The model under review builds one solid part; all positions refer to its coordinate system, in mm. A direction names the side the tool comes from. Coordinates: 2 decimals unless noted, no trailing zeros. Write each loop counter-clockwise with the first axis right and the second up, starting at its lowest first coordinate (ties: lowest second). Pieces come first, ordered by that corner, then holes.
```python
from build123d import *

# Parameters (mm, degrees)
F0_W         = 85
F0_H         = 44
F1_DEPTH     = 28
F2_W         = 49
F2_H         = 37
F3_DEPTH     = 9
F2_W_2       = 25
F2_H_2       = 42
F4_DEPTH     = 7.5
F5_W         = 25
F5_H         = 13
F5_R         = 1.25
F6_DEPTH     = 16
F7_T1_DEPTH  = 22
F7_T3_DEPTH  = 32.5
F7_T5_DEPTH  = 79
F7_T7_DEPTH  = 38
F7_T9_DEPTH  = 68
F7_T11_DEPTH = 89.5
F7_T13_DEPTH = 48.5
F7_S17_W     = 3
F7_S17_H     = 3
F7_T18_DEPTH = 3
F7_S23_W     = 3
F7_S23_H     = 3
F7_T24_DEPTH = 3
F7_S29_W     = 3
F7_S29_H     = 3
F7_T30_DEPTH = 3
F7_S35_W     = 3
F7_S35_H     = 3
F7_T36_DEPTH = 3
F7_S41_W     = 3
F7_S41_H     = 3
F7_T42_DEPTH = 3


# Not quite as in the source:
# - a fillet or chamfer that OpenCascade refuses, or shapes differently, is made with other operations: its cross-section is extruded or revolved along the edge and cut away or added


with BuildPart() as f1:
    # F0 (on Top) → F1 (new body)
    with BuildSketch(Plane.XY):
        with Locations((12.7505162358, -9.2363715138)):
            Rectangle(F0_W, F0_H)
    extrude(amount=F1_DEPTH)

    # F2 (on face) → F3 (cut)
    with BuildSketch(Plane.XY.offset(28)):
        with Locations((-3.2494837642, -9.2363715138)):
            Rectangle(F2_W, F2_H)
    extrude(amount=-F3_DEPTH, mode=Mode.SUBTRACT)

    # F2 (on face) → F4 (cut)
    with BuildSketch(Plane.XY.offset(28)):
        with Locations((35.7505162358, -8.2363715138)):
            Rectangle(F2_W_2, F2_H_2)
    extrude(amount=-F4_DEPTH, mode=Mode.SUBTRACT)

    # F5 (on face) → F6 (cut)
    with BuildSketch(Plane(origin=(0, 0, 0), x_dir=(1, 0, 0), z_dir=(0, 0, -1))):
        with Locations((-12.2494837642, 9.2363715138)):
            Rectangle(F5_W, F5_H)
        with Locations((37.7505162358, 9.2363715138)):
            Rectangle(F5_W, F5_H)
        with Locations((-26.9994837642, 9.2363715138)):
            Circle(F5_R)
        with Locations((2.5005162358, 9.2363715138)):
            Circle(F5_R)
        with Locations((23.0005162358, 9.2363715138)):
            Circle(F5_R)
        with Locations((52.5005162358, 9.2363715138)):
            Circle(F5_R)
    extrude(amount=-F6_DEPTH, mode=Mode.SUBTRACT)

    # F7: fillet of radius 3 on 11 edges, made by hand

    # F7_s2 → F7_t1 (cut)
    with BuildSketch(Plane.XY.offset(3)):
        with BuildLine():
            ThreePointArc((55.2505162358, -28.2363715138), (54.3718365794, -30.3576918574), (52.2505162358, -31.2363715138))
            Line((52.2505162358, -31.2363715138), (55.2505162358, -31.2363715138))
            Line((55.2505162358, -31.2363715138), (55.2505162358, -28.2363715138))
        make_face()
    extrude(amount=F7_T1_DEPTH, mode=Mode.SUBTRACT)

    # F7_s4 → F7_t3 (cut)
    with BuildSketch(Plane.XY.offset(3)):
        with BuildLine():
            ThreePointArc((52.2505162358, 12.7636284862), (54.3718365794, 11.8849488297), (55.2505162358, 9.7636284862))
            Line((55.2505162358, 9.7636284862), (55.2505162358, 12.7636284862))
            Line((55.2505162358, 12.7636284862), (52.2505162358, 12.7636284862))
        make_face()
        with BuildLine():
            ThreePointArc((-29.7494837642, -28.2363715138), (-28.8708041077, -30.3576918574), (-26.7494837642, -31.2363715138))
            Line((-26.7494837642, -31.2363715138), (-29.7494837642, -31.2363715138))
            Line((-29.7494837642, -31.2363715138), (-29.7494837642, -28.2363715138))
        make_face()
        with BuildLine():
            ThreePointArc((-26.7494837642, 12.7636284862), (-28.8708041077, 11.8849488297), (-29.7494837642, 9.7636284862))
            Line((-29.7494837642, 9.7636284862), (-29.7494837642, 12.7636284862))
            Line((-29.7494837642, 12.7636284862), (-26.7494837642, 12.7636284862))
        make_face()
    extrude(amount=F7_T3_DEPTH, mode=Mode.SUBTRACT)

    # F7_s6 → F7_t5 (cut)
    with BuildSketch(Plane.YZ.offset(-26.7494837642)):
        with BuildLine():
            ThreePointArc((12.7636284862, 3), (11.8849488297, 0.8786796564), (9.7636284862, 0))
            Line((9.7636284862, 0), (12.7636284862, 0))
            Line((12.7636284862, 0), (12.7636284862, 3))
        make_face()
        with BuildLine():
            ThreePointArc((-28.2363715138, 0), (-30.3576918574, 0.8786796564), (-31.2363715138, 3))
            Line((-31.2363715138, 3), (-31.2363715138, 0))
            Line((-31.2363715138, 0), (-28.2363715138, 0))
        make_face()
    extrude(amount=F7_T5_DEPTH, mode=Mode.SUBTRACT)

    # F7_s8 → F7_t7 (cut)
    with BuildSketch(Plane.XZ.offset(-9.7636284862)):
        with BuildLine():
            ThreePointArc((-26.7494837642, 0), (-28.8708041077, 0.8786796564), (-29.7494837642, 3))
            Line((-29.7494837642, 3), (-29.7494837642, 0))
            Line((-29.7494837642, 0), (-26.7494837642, 0))
        make_face()
        with BuildLine():
            ThreePointArc((52.2505162358, 0), (54.3718365794, 0.8786796564), (55.2505162358, 3))
            Line((55.2505162358, 3), (55.2505162358, 0))
            Line((55.2505162358, 0), (52.2505162358, 0))
        make_face()
    extrude(amount=F7_T7_DEPTH, mode=Mode.SUBTRACT)

    # F7_s10 → F7_t9 (cut)
    with BuildSketch(Plane.YZ.offset(-37.2494837642)):
        with BuildLine():
            ThreePointArc((12.7636284862, 25), (11.8849488297, 27.1213203436), (9.7636284862, 28))
            Line((9.7636284862, 28), (12.7636284862, 28))
            Line((12.7636284862, 28), (12.7636284862, 25))
        make_face()
    extrude(amount=F7_T9_DEPTH, mode=Mode.SUBTRACT)

    # F7_s12 → F7_t11 (cut)
    with BuildSketch(Plane.YZ.offset(-37.2494837642)):
        with BuildLine():
            ThreePointArc((-28.2363715138, 28), (-30.3576918574, 27.1213203436), (-31.2363715138, 25))
            Line((-31.2363715138, 25), (-31.2363715138, 28))
            Line((-31.2363715138, 28), (-28.2363715138, 28))
        make_face()
    extrude(amount=F7_T11_DEPTH, mode=Mode.SUBTRACT)

    # F7_s14 → F7_t13 (cut)
    with BuildSketch(Plane.XZ.offset(-20.2636284862)):
        with BuildLine():
            ThreePointArc((52.2505162358, 28), (54.3718365794, 27.1213203436), (55.2505162358, 25))
            Line((55.2505162358, 25), (55.2505162358, 28))
            Line((55.2505162358, 28), (52.2505162358, 28))
        make_face()
    extrude(amount=F7_T13_DEPTH, mode=Mode.SUBTRACT)


with BuildPart() as f7_tool16:
    # F7_s17 → F7_t18 (new body)
    with BuildSketch(Plane.XZ.offset(28.2363715138)):
        with Locations((53.7505162358, 1.5)):
            Rectangle(F7_S17_W, F7_S17_H)
    extrude(amount=F7_T18_DEPTH)

    # F7_s19 → F7_t20 (revolve, cut)
    with BuildSketch(Plane(origin=(52.2505162358, -28.2363715138, 3), x_dir=(-0.7071067812, 0, 0.7071067812), z_dir=(0.7071067812, 0, 0.7071067812))):
        with BuildLine():
            ThreePointArc((0, -3), (3, 0), (0, 3))
            Line((0, 3), (0, -3))
        make_face()
    revolve(axis=Axis((52.2505162358, -28.2363715138, 3), (0, -1, 0)), mode=Mode.SUBTRACT)


with BuildPart() as f1_1:
    add(f1.part)

    # F7_t15: cut F7_tool16
    add(f7_tool16.part, mode=Mode.SUBTRACT)


with BuildPart() as f7_tool22:
    # F7_s23 → F7_t24 (new body)
    with BuildSketch(Plane.XZ.offset(28.2363715138)):
        with Locations((53.7505162358, 26.5)):
            Rectangle(F7_S23_W, F7_S23_H)
    extrude(amount=F7_T24_DEPTH)

    # F7_s25 → F7_t26 (revolve, cut)
    with BuildSketch(Plane(origin=(52.2505162358, -28.2363715138, 25), x_dir=(-0.7071067812, 0, -0.7071067812), z_dir=(-0.7071067812, 0, 0.7071067812))):
        with BuildLine():
            ThreePointArc((0, -3), (3, 0), (0, 3))
            Line((0, 3), (0, -3))
        make_face()
    revolve(axis=Axis((52.2505162358, -28.2363715138, 25), (0, -1, 0)), mode=Mode.SUBTRACT)


with BuildPart() as f1_2:
    add(f1_1.part)

    # F7_t21: cut F7_tool22
    add(f7_tool22.part, mode=Mode.SUBTRACT)


with BuildPart() as f7_tool28:
    # F7_s29 → F7_t30 (new body)
    with BuildSketch(Plane.XZ.offset(-9.7636284862)):
        with Locations((53.7505162358, 1.5)):
            Rectangle(F7_S29_W, F7_S29_H)
    extrude(amount=-F7_T30_DEPTH)

    # F7_s31 → F7_t32 (revolve, cut)
    with BuildSketch(Plane(origin=(52.2505162358, 9.7636284862, 3), x_dir=(-0.7071067812, 0, 0.7071067812), z_dir=(-0.7071067812, 0, -0.7071067812))):
        with BuildLine():
            ThreePointArc((0, -3), (3, 0), (0, 3))
            Line((0, 3), (0, -3))
        make_face()
    revolve(axis=Axis((52.2505162358, 9.7636284862, 3), (0, 1, 0)), mode=Mode.SUBTRACT)


with BuildPart() as f1_3:
    add(f1_2.part)

    # F7_t27: cut F7_tool28
    add(f7_tool28.part, mode=Mode.SUBTRACT)


with BuildPart() as f7_tool34:
    # F7_s35 → F7_t36 (new body)
    with BuildSketch(Plane.XZ.offset(28.2363715138)):
        with Locations((-28.2494837642, 1.5)):
            Rectangle(F7_S35_W, F7_S35_H)
    extrude(amount=F7_T36_DEPTH)

    # F7_s37 → F7_t38 (revolve, cut)
    with BuildSketch(Plane(origin=(-26.7494837642, -28.2363715138, 3), x_dir=(0.7071067812, 0, 0.7071067812), z_dir=(0.7071067812, 0, -0.7071067812))):
        with BuildLine():
            ThreePointArc((0, -3), (3, 0), (0, 3))
            Line((0, 3), (0, -3))
        make_face()
    revolve(axis=Axis((-26.7494837642, -28.2363715138, 3), (0, -1, 0)), mode=Mode.SUBTRACT)


with BuildPart() as f1_4:
    add(f1_3.part)

    # F7_t33: cut F7_tool34
    add(f7_tool34.part, mode=Mode.SUBTRACT)


with BuildPart() as f7_tool40:
    # F7_s41 → F7_t42 (new body)
    with BuildSketch(Plane.XZ.offset(-9.7636284862)):
        with Locations((-28.2494837642, 1.5)):
            Rectangle(F7_S41_W, F7_S41_H)
    extrude(amount=-F7_T42_DEPTH)

    # F7_s43 → F7_t44 (revolve, cut)
    with BuildSketch(Plane(origin=(-26.7494837642, 9.7636284862, 3), x_dir=(0.7071067812, 0, 0.7071067812), z_dir=(-0.7071067812, 0, 0.7071067812))):
        with BuildLine():
            ThreePointArc((0, -3), (3, 0), (0, 3))
            Line((0, 3), (0, -3))
        make_face()
    revolve(axis=Axis((-26.7494837642, 9.7636284862, 3), (0, 1, 0)), mode=Mode.SUBTRACT)


with BuildPart() as f1_5:
    add(f1_4.part)

    # F7_t39: cut F7_tool40
    add(f7_tool40.part, mode=Mode.SUBTRACT)


solid = f1_5.part
```
Item 1: Mouldability with a two-part tool opening along X and no side actions: class faces 5 (the face through (54.348, -7.449, 27.145)), 6 (the face through (53.08, -8.13, 7.89)), 7 (the face through (-24.749, -9, 8)), 8 (the face through (12.198, -30.334, 0.855)) as pulls with the +X half, pulls with the -X half, needs draft (parallel to the pull), parting line crosses it, or undercut.
Solved:
face 5: pulls with the +X half
face 6: undercut
face 7: undercut
face 8: needs draft
Item 2: Take a section at A-A, the plane y = -12.5. Write out the cut boundary in (x, z), plus the area to 3 significant figures.
Solved:
outline: (-29.75, 3) arc R3 ccw to (-26.75, 0) - (-24.75, 0) - (-24.75, 16) - (0.25, 16) - (0.25, 0) - (25.25, 0) - (25.25, 16) - (50.25, 16) - (50.25, 0) - (52.25, 0) arc R3 ccw to (55.25, 3) - (55.25, 25) arc R3 ccw to (52.25, 28) - (48.25, 28) - (48.25, 20.5) - (23.25, 20.5) - (23.25, 28) - (21.25, 28) - (21.25, 19) - (-27.75, 19) - (-27.75, 28) - (-29.75, 28) - close
area: 946 mm2
Item 3: For pin 1 (2 mm diameter, centred on x = 28, y = -1.5, fed in from +Z); pin 2 (6 mm diameter, centred on x = 16, y = -16, fed in from +Z); pin 3 (3 mm diameter, centred on x = -5, y = -7, fed in from -Z), all flat-tipped, find the tip position at first contact; note any pin that passes through.
Solved:
pin 1: stops at z = 20.5
pin 2: stops at z = 19
pin 3: stops at z = 16
Item 4: Machinability: for faces 1 (the face through (22.73, -8.016, 7.888)), 2 (the face through (21.251, -9, 24)), 3 (the face through (48.251, -9, 24)), 4 (the face through (12, -9, 0)), which of the approach directions +Z, -Z, +X, -X, +Y, -Y give a long, thin tool a straight path to every point of the face, cutting with its end or side? Answer none if there is none.
Solved:
face 1: -Z
face 2: +Z
face 3: +Z, +Y
face 4: -Z, +X, -X, +Y, -Y
Item 5: To check wall thickness, follow line 1 along X through (y, z) = (5, 22); line 2 along X through (y, z) = (-13.5, 11); line 3 along Y through (x, z) = (29, 11.25). State the ranges of each line that lie inside material, in increasing order.
Solved:
line 1: x = -29.75 to -27.75, 21.25 to 23.25, 48.25 to 55.25
line 2: x = -29.75 to -24.75, 0.25 to 25.25, 50.25 to 55.25
line 3: y = -31.24 to -15.74, -2.74 to 12.76
Item 6: Take a section at D-D, the plane y = 7.5. Write out the cut boundary in (x, z).
Solved:
outline: (-29.75, 3) arc R3 ccw to (-26.75, 0) - (52.25, 0) arc R3 ccw to (55.25, 3) - (55.25, 25) arc R3 ccw to (52.25, 28) - (48.25, 28) - (48.25, 20.5) - (23.25, 20.5) - (23.25, 28) - (21.25, 28) - (21.25, 19) - (-27.75, 19) - (-27.75, 28) - (-29.75, 28) - close
Item 7: Take a section at B-B, the plane x = 14. Write out the cut boundary in (y, z).
Solved:
outline: (-31.24, 3) arc R3 ccw to (-28.24, 0) - (9.76, 0) arc R3 ccw to (12.76, 3) - (12.76, 25) arc R3 ccw to (9.76, 28) - (9.26, 28) - (9.26, 19) - (-27.74, 19) - (-27.74, 28) - (-28.24, 28) arc R3 ccw to (-31.24, 25) - close
Item 8: Take a section at C-C, the plane z = 9.5. Write out the cut boundary in (x, y), plus the area to 3 significant figures.
Solved:
outline: (-29.75, -28.24) arc R3 ccw to (-26.75, -31.24) - (52.25, -31.24) arc R3 ccw to (55.25, -28.24) - (55.25, 9.76) arc R3 ccw to (52.25, 12.76) - (-26.75, 12.76) arc R3 ccw to (-29.75, 9.76) - close; hole circle Ø2.5 at (-27, -9.24); hole (-24.75, -15.74) - (0.25, -15.74) - (0.25, -2.74) - (-24.75, -2.74) - close; hole circle Ø2.5 at (2.5, -9.24); hole circle Ø2.5 at (23, -9.24); hole (25.25, -15.74) - (50.25, -15.74) - (50.25, -2.74) - (25.25, -2.74) - close; hole circle Ø2.5 at (52.5, -9.24)
area: 3,060 mm2
